```python
from build123d import *

# Parameters (mm, degrees)
SKETCH1_R           = 70
SKETCH1_R_2         = 3.175
BOSS_EXTRUDE2_DEPTH = 5
SKETCH2_R           = 5
SKETCH2_R_2         = 3.175
BOSS_EXTRUDE4_DEPTH = 15
SKETCH3_R           = 2
CUT_EXTRUDE1_DEPTH  = 10


with BuildPart() as part:
    # Sketch1 → Boss-Extrude2 (new body)
    with BuildSketch(Plane(origin=(0, 0, 0), x_dir=(1, 0, 0), z_dir=(0, 1, 0))):
        with Locations(Location((0, 0, 0), (0, 0, 270))):
            Circle(SKETCH1_R)
        with Locations(Location((0, 0, 0), (0, 0, 270))):
            Circle(SKETCH1_R_2, mode=Mode.SUBTRACT)
    extrude(amount=BOSS_EXTRUDE2_DEPTH)

    # Sketch2 → Boss-Extrude4 (add)
    with BuildSketch(Plane(origin=(0, 5, 0), x_dir=(1, 0, 0), z_dir=(0, 1, 0))):
        with Locations(Location((0, 0, 0), (0, 0, 270))):
            Circle(SKETCH2_R)
        with Locations(Location((0, 0, 0), (0, 0, 270))):
            Circle(SKETCH2_R_2, mode=Mode.SUBTRACT)
    extrude(amount=BOSS_EXTRUDE4_DEPTH)

    # Sketch3 → Cut-Extrude1 (cut)
    with BuildSketch(Plane(origin=(0, 5, 0), x_dir=(1, 0, 0), z_dir=(0, 1, 0))):
        with Locations(Location((-17.267766953, 48.267766953, 0), (0, 0, 270))):
            Circle(SKETCH3_R)
        with Locations(Location((17.267766953, 48.267766953, 0), (0, 0, 270))):
            Circle(SKETCH3_R)
        with Locations(Location((-17.267766953, 18.732233047, 0), (0, 0, 270))):
            Circle(SKETCH3_R)
        with Locations(Location((17.267766953, 18.732233047, 0), (0, 0, 270))):
            Circle(SKETCH3_R)
    extrude(amount=-CUT_EXTRUDE1_DEPTH, mode=Mode.SUBTRACT)


solid = part.part
```
Read the model definition and answer for the solid it produces. Units are mm, in the model's axes. A direction names the side the tool comes from. Coordinates: 2 decimals unless noted, no trailing zeros. Write each loop counter-clockwise with the first axis right and the second up, starting at its lowest first coordinate (ties: lowest second). Pieces come first, ordered by that corner, then holes. Notation, with made-up numbers: (11.25, 85) -> (49.25, 85) arc R24 ccw to (49.25, 118) -> close; hole circle Ø1 at (-22, 37). An arc over 180 degrees is marked (long way). Answer as a JSON object with one key per item and string values.
Q1. Consider line 1 (X direction, y = 15.75, z = 0) (3 decimals); line 2 (X direction, y = 4.25, z = -20.5); line 3 (Y direction, x = 6.5, z = -62.5). Determine where each line is inside the solid, lowest interval first. Write a range as [from, to].
The answers:
{"line 1": "x = [-5, -3.175], [3.175, 5]", "line 2": "x = [-66.93, -18.2], [-16.33, 16.33], [18.2, 66.93]", "line 3": "y = [0, 5]"}
Q2. Flat-ended cylindrical pins translate along their axes: pin 1 Ø12 at (x, y) = (9, 5.5) entering from +Z; pin 2 Ø12 at (x, z) = (52.5, -27.5) entering from +Y; pin 3 Ø12 at (x, y) = (-1, 12.5) entering from -Z; pin 4 Ø4.5 at (x, z) = (17.27, -48.27) entering from -Y. Find the tip coordinate at first contact, or state that the pin passes through.
The answers:
{"pin 1": "stops at z = 69.93", "pin 2": "stops at y = 5", "pin 3": "stops at z = -5", "pin 4": "stops at y = 0"}
Q3. A tool of negligible diameter and unlimited length cuts with its end or side. For faces 1 (the cylindrical face through (-1.93, 9.86, -2.52)), 2 (the cylindrical face through (-4.88, 12.4, -1.08)), from which of +Z, -Z, +X, -X, +Y, -Y can it reach the whole face along a straight path? Write none if from no direction.
The answers:
{"face 1": "+Y, -Y", "face 2": "+Y"}
Q4. The part is cut by section D-D on z = -30. Give the vertices of the cut face in (x, y), then the cut area to 3 significant figures.
The answers:
{"outline": "(-63.25, 0) -> (63.25, 0) -> (63.25, 5) -> (-63.25, 5) -> close", "area": "632 mm2"}
Q5. The part is cut by section C-C on y = 8.75. Give the vertices of the cut face in (x, z) (3 decimals).
The answers:
{"outline": "circle Ø10 at (0, 0); hole circle Ø6.35 at (0, 0)"}
Q6. The part is cut by section B-B on x = 0. Give the vertices of the cut face in (y, z) (3 decimals), then the cut area to 3 significant figures.
The answers:
{"outline": "(0, -70) -> (5, -70) -> (5, -5) -> (20, -5) -> (20, -3.175) -> (0, -3.175) -> close; (0, 3.175) -> (20, 3.175) -> (20, 5) -> (5, 5) -> (5, 70) -> (0, 70) -> close", "area": "723 mm2"}
Q7. Determine the mould class of faces 3 (the cylindrical face through (-18.034, 2.535, -16.885)), 4 (the cylindrical face through (-42.594, 2.465, -55.55)), 5 (the flat face through (-1, 20, 3.3)) for opening direction X: pulls with the +X half, pulls with the -X half, needs draft (parallel to the pull), parting line crosses it, or undercut.
The answers:
{"face 3": "undercut", "face 4": "parting line crosses it", "face 5": "needs draft"}
Q8. The part is cut by section A-A on z = 0. Give the vertices of the cut face in (x, y) (3 decimals), then the cut area to 3 significant figures.
The answers:
{"outline": "(-70, 0) -> (-3.175, 0) -> (-3.175, 20) -> (-5, 20) -> (-5, 5) -> (-70, 5) -> close; (3.175, 0) -> (70, 0) -> (70, 5) -> (5, 5) -> (5, 20) -> (3.175, 20) -> close", "area": "723 mm2"}
